```python
from build123d import *

# Parameters (mm, degrees)
F0_W     = 185.310639
F0_H     = 100.29944
F1_DEPTH = 43.18
F2_W     = 142.667748
F2_H     = 63.255836
F3_DEPTH = 25.4
F4_R     = 5.08


with BuildPart() as f1:
    # F0 (on Top) → F1 (new body)
    with BuildSketch(Plane.XY):
        with Locations((10.269184, 4.973244)):
            Rectangle(F0_W, F0_H)
    extrude(amount=F1_DEPTH)

    # F2 (on face) → F3 (cut)
    with BuildSketch(Plane.XY.offset(43.18)):
        with Locations((14.403265, 9.399725)):
            Rectangle(F2_W, F2_H)
    extrude(amount=-F3_DEPTH, mode=Mode.SUBTRACT)

    # F4
    f4_edges = [f1.edges().sort_by_distance(p)[0] for p in [
        (-82.386136, -45.176476, 21.59),
        (102.924503, -45.176476, 21.59),
        (102.924503, 55.122964, 21.59),
        (10.269184, 55.122964, 43.18),
        (14.403265, 41.027643, 43.18),
        (-82.386136, 55.122964, 21.59),
        (-56.930609, 41.027643, 30.48),
        (14.403265, -22.228193, 43.18),
        (14.403265, 41.027643, 17.78),
        (-56.930609, 9.399725, 43.18),
        (-56.930609, 9.399725, 17.78),
        (10.269184, 55.122964, 0),
        (-82.386136, 4.973244, 43.18),
        (-82.386136, 4.973244, 0),
    ]]
    fillet(f4_edges, radius=F4_R)


solid = f1.part
```
The listing builds one solid part. Answer for the finished solid, in the listing's coordinates (mm). A direction names the side the tool comes from. Coordinates: 2 decimals unless noted, no trailing zeros. Write each loop counter-clockwise with the first axis right and the second up, starting at its lowest first coordinate (ties: lowest second). Pieces come first, ordered by that corner, then holes. Notation, with made-up numbers: (-32.5, -19.5) -> (10.5, -19.5) arc R29 cw to (10.5, 16.5) -> close; hole circle Ø8 at (-5, -6). An arc over 180 degrees is marked (long way). Write each question's results on one line, items separated by ' | '. Start each with the question number.
1) For a pull along Y with two mould halves and no side action, classify faces 3 (the flat face through (-56.931, 6, 31)), 4 (the cylindrical face through (-80.938, -43.649, 21.892)), 5 (the flat face through (12, -29, 43.18)) as +Y half, -Y half, draft (parallel to the pull), parting line (faces both ways), or undercut.
2) Straight lines are drawn through the part: probe 1 along X at (y, z) = (10, 31); probe 2 along Y at (x, z) = (20.5, 32); probe 3 along Z at (x, y) = (32.5, 19). For each, find the intervals that lie inside material, in ascending order.
3) A cutting plane is placed at D-D (z = 20.5). Determine the outline of the cut face in (x, y), then the cut area to 3 significant figures.
4) A cutting plane is placed at C-C (x = -37.5). Determine the outline of the cut face in (y, z).
5) A tool of negligible diameter and unlimited length cuts with its end or side. For faces 1 (the flat face through (16, 7, 17.78)), 2 (the cylindrical face through (101.397, -43.728, 21.892)), from which of +Z, -Z, +X, -X, +Y, -Y can it reach the whole face along a straight path? Write none if from no direction.
6) A cutting plane is placed at B-B (y = -16). Determine the outline of the cut face in (x, z).
7) A cutting plane is placed at A-A (z = 30.5). Determine the outline of the cut face in (x, y), then the cut area to 3 significant figures.
Values follow:
1) face 3: undercut | face 4: -Y half | face 5: draft
2) probe 1: -82.39 to -56.93, 85.74 to 102.92 | probe 2: -45.18 to -22.23, 41.03 to 55.12 | probe 3: 0 to 17.78
3) outline: (-82.39, -40.1) arc R5.08 ccw to (-77.31, -45.18) -> (97.84, -45.18) arc R5.08 ccw to (102.92, -40.1) -> (102.92, 50.04) arc R5.08 ccw to (97.84, 55.12) -> (-77.31, 55.12) arc R5.08 ccw to (-82.39, 50.04) -> close; hole (-56.35, -22.23) -> (85.74, -22.23) -> (85.74, 40.45) -> (-51.85, 40.45) arc R4.5 ccw to (-56.35, 35.95) -> close | area: 9,660 mm²
4) outline: (-45.18, 0) -> (50.04, 0) arc R5.08 ccw to (55.12, 5.08) -> (55.12, 38.1) arc R5.08 ccw to (50.04, 43.18) -> (46.11, 43.18) arc R5.08 ccw to (41.03, 38.1) -> (41.03, 22.86) arc R5.08 cw to (35.95, 17.78) -> (-22.23, 17.78) -> (-22.23, 38.1) arc R5.08 ccw to (-27.31, 43.18) -> (-45.18, 43.18) -> close
5) face 1: +Z | face 2: +Z, -Z, +X, -Y
6) outline: (-82.39, 5.08) arc R5.08 ccw to (-77.31, 0) -> (102.92, 0) -> (102.92, 43.18) -> (85.74, 43.18) -> (85.74, 17.78) -> (-51.85, 17.78) arc R5.08 cw to (-56.93, 22.86) -> (-56.93, 38.1) arc R5.08 ccw to (-62.01, 43.18) -> (-77.31, 43.18) arc R5.08 ccw to (-82.39, 38.1) -> close
7) outline: (-82.39, -40.1) arc R5.08 ccw to (-77.31, -45.18) -> (97.84, -45.18) arc R5.08 ccw to (102.92, -40.1) -> (102.92, 50.04) arc R5.08 ccw to (97.84, 55.12) -> (-77.31, 55.12) arc R5.08 ccw to (-82.39, 50.04) -> close; hole (-56.93, -22.23) -> (85.74, -22.23) -> (85.74, 41.03) -> (-51.85, 41.03) arc R5.08 ccw to (-56.93, 35.95) -> close | area: 9,550 mm²
